from build123d import *

# Parameters (mm, degrees)
EXTRUDE_1_DEPTH     = 24
SKETCH_2_W          = 46
SKETCH_2_H          = 21.081573772
EXTRUDE_2_DEPTH     = 3
SKETCH_3_W          = 46
SKETCH_3_H          = 21.081573772
EXTRUDE_3_DEPTH     = 3
SKETCH_6_R          = 5
CUT_EXTRUDE_2_DEPTH = 10
SKETCH_7_R          = 3
CUT_EXTRUDE_3_DEPTH = 10


with BuildPart() as part:
    # 草图1 → 凸台-拉伸1 (new body)
    with BuildSketch(Plane.XY):
        Polygon((-66, 28.893533875), (-43, 28.893533875), (-43, 10.811960103), (-3, 10.811960103), (-3, 28.893533875), (20, 28.893533875), (20, 25.893533875), (0, 25.893533875), (0, 7.811960103), (-46, 7.811960103), (-46, 25.893533875), (-66, 25.893533875), align=None)
    extrude(amount=EXTRUDE_1_DEPTH)

    # 草图2 → 凸台-拉伸2 (add)
    with BuildSketch(Plane.XY.offset(24)):
        with Locations((-23, 18.352746989)):
            Rectangle(SKETCH_2_W, SKETCH_2_H)
    extrude(amount=EXTRUDE_2_DEPTH)

    # 草图3 → 凸台-拉伸3 (add)
    with BuildSketch(Plane(origin=(0, 0, 0), x_dir=(-1, 0, 0), z_dir=(0, 0, -1))):
        with Locations((23, 18.352746989)):
            Rectangle(SKETCH_3_W, SKETCH_3_H)
    extrude(amount=EXTRUDE_3_DEPTH)

    # 草图6 → 切除-拉伸2 (cut)
    with BuildSketch(Plane.ZY.offset(46)):
        with Locations((12.093557596, 17.339206361)):
            Circle(SKETCH_6_R)
    extrude(amount=-CUT_EXTRUDE_2_DEPTH, mode=Mode.SUBTRACT)

    # 草图7 → 切除-拉伸3 (cut)
    with BuildSketch(Plane.XZ.offset(-25.893533875)):
        with Locations((10, 12)):
            Circle(SKETCH_7_R)
        with Locations((-56, 12)):
            Circle(SKETCH_7_R)
    extrude(amount=-CUT_EXTRUDE_3_DEPTH, mode=Mode.SUBTRACT)


solid = part.part
Input: part model. Units: mm. Frame: model coordinates. A direction names the side the tool comes from. Give positions to 0.01 mm unless a question says otherwise; leave off trailing zeros. Write each loop counter-clockwise with the first axis right and the second up, starting at its lowest first coordinate (ties: lowest second). Pieces come first, ordered by that corner, then holes. Notation, with made-up numbers: M 28,24.5 L 84,24.5 A31 cw 84,60.5 Z; hole C 59.25,54.5 d5. An arc over 180 degrees is marked long. Use one line per item in the form item = value.
1. Cut plane D-D on x = -27. Return loops of the section in (y, z).
Outcome:
outline = M 7.81,-3 L 28.89,-3 L 28.89,0 L 10.81,0 L 10.81,24 L 28.89,24 L 28.89,27 L 7.81,27 Z
2. Cut plane C-C on z = 12. Return loops of the section in (x, y).
Outcome:
outline = M -66,25.89 L -59,25.89 L -59,28.89 L -66,28.89 Z; M -53,25.89 L -46,25.89 L -46,22.34 L -43,22.34 L -43,28.89 L -53,28.89 Z; M -46,7.81 L 0,7.81 L 0,25.89 L 7,25.89 L 7,28.89 L -3,28.89 L -3,10.81 L -43,10.81 L -43,12.34 L -46,12.34 Z; M 13,25.89 L 20,25.89 L 20,28.89 L 13,28.89 Z
3. Mould query, pull axis X, two halves, no side actions, for faces 1 (the face through (20, 27, 12)), 2 (the face through (-22, 28.894, -1)), 3 (the face through (-59, 27, 12)). Classes: released by +X, released by -X, zero draft, split by the parting line, or undercut.
Outcome:
face_1 = released by +X
face_2 = zero draft
face_3 = undercut
4. Cut plane A-A on x = -56. Return loops of the section in (y, z).
Outcome:
outline = M 25.89,0 L 28.89,0 L 28.89,9 L 25.89,9 Z; M 25.89,15 L 28.89,15 L 28.89,24 L 25.89,24 Z
5. First-contact query: P1, Ø10, axis at x = 14.5, z = 9.5, coming from the -Y side; P2, Ø1.5, axis at x = -42, z = 12.5, coming from the +Y side; P3, Ø3.5, axis at x = -60, y = 27.5, coming from the -Z side. Flat tips, straight axial feed; report the tip coordinate or a pass-through.
Outcome:
P1 = 25.89
P2 = 10.81
P3 = 0
6. Reachability of faces 4 (the face through (-3, 20, 12)), 5 (the face through (10, 27, 24)), 6 (the face through (-58, 25.894, 9)), 7 (the face through (10, 27, 0)), 8 (the face through (12, 25.894, 9)) from +Z, -Z, +X, -X, +Y, -Y: full face, straight path, thin tool, end or side. Return the list, or none.
Outcome:
face_4 = +Y
face_5 = +Z, +X, +Y, -Y
face_6 = +Z, -Z, -X, -Y
face_7 = -Z, +X, +Y, -Y
face_8 = +Z, -Z, +X, -Y
7. Ray query, L1, parallel to Z at x = -5, y = 26; L2, parallel to Z at x = -56, y = 26.7; L3, parallel to X at y = 21.25, z = 5.5. Return the intervals inside material, ascending.
Outcome:
L1 = -3 to 0, 24 to 27
L2 = 0 to 9, 15 to 24
L3 = -46 to -43, -3 to 0
8. Cut plane B-B on z = 2.5. Return loops of the section in (x, y).
Outcome:
outline = M -66,25.89 L -46,25.89 L -46,7.81 L 0,7.81 L 0,25.89 L 20,25.89 L 20,28.89 L -3,28.89 L -3,10.81 L -43,10.81 L -43,28.89 L -66,28.89 Z
